```python
from build123d import *

# Parameters (mm, degrees)
BOSS_EXTRUDE1_DEPTH = 10
CUT_EXTRUDE1_DEPTH  = 10
SKETCH3_R           = 2.5
CUT_EXTRUDE2_DEPTH  = 7


with BuildPart() as part:
    # Sketch1 → Boss-Extrude1 (new body)
    with BuildSketch(Plane(origin=(0, 0, 0), x_dir=(1, 0, 0), z_dir=(0, 1, 0))):
        with BuildLine():
            Line((-40, 50), (40, 50))
            ThreePointArc((40, 50), (47.071067812, 47.071067812), (50, 40))
            Line((50, 40), (50, -40))
            ThreePointArc((50, -40), (47.071067812, -47.071067812), (40, -50))
            Line((40, -50), (-40, -50))
            ThreePointArc((-40, -50), (-47.071067812, -47.071067812), (-50, -40))
            Line((-50, -40), (-50, 40))
            ThreePointArc((-50, 40), (-47.071067812, 47.071067812), (-40, 50))
        make_face()
    extrude(amount=BOSS_EXTRUDE1_DEPTH)

    # Sketch2 → Cut-Extrude1 (cut)
    with BuildSketch(Plane(origin=(0, 10, 0), x_dir=(1, 0, 0), z_dir=(0, 1, 0))):
        with BuildLine():
            Line((-30, -40), (30, -40))
            ThreePointArc((30, -40), (37.071067812, -37.071067812), (40, -30))
            Line((40, -30), (40, 30))
            ThreePointArc((40, 30), (37.071067812, 37.071067812), (30, 40))
            Line((30, 40), (-30, 40))
            ThreePointArc((-30, 40), (-37.071067812, 37.071067812), (-40, 30))
            Line((-40, 30), (-40, -30))
            ThreePointArc((-40, -30), (-37.071067812, -37.071067812), (-30, -40))
        make_face()
    extrude(amount=-CUT_EXTRUDE1_DEPTH, mode=Mode.SUBTRACT)

    # Sketch3 → Cut-Extrude2 (cut)
    with BuildSketch(Plane(origin=(0, 10, 0), x_dir=(1, 0, 0), z_dir=(0, 1, 0))):
        with Locations(Location((-42, 42, 0), (0, 0, 270))):
            Circle(SKETCH3_R)
        with Locations(Location((42, 42, 0), (0, 0, 270))):
            Circle(SKETCH3_R)
        with Locations(Location((42.000013816, -42, 0), (0, 0, 270))):
            Circle(SKETCH3_R)
        with Locations(Location((-41.999986184, -42, 0), (0, 0, 270))):
            Circle(SKETCH3_R)
    extrude(amount=-CUT_EXTRUDE2_DEPTH, mode=Mode.SUBTRACT)


solid = part.part
```
Input: part model. Units: mm. Frame: model coordinates. A direction names the side the tool comes from. Coordinates: 2 decimals unless noted, no trailing zeros. Loops run counter-clockwise (first coordinate to the right, second up) from the corner with the lowest first, then second, coordinate; pieces in that order, holes last. Notation, with made-up numbers: M 36.25,-39.5 L 91.25,-39.5 A29 ccw 91.25,-19.5 Z; hole C 87.5,21.5 d6. An arc over 180 degrees is marked long. Use a Markdown table: item, result. Add a question column.
1) Section B-B, the plane z = -6.5. Return the cut outline in (x, y).
2) Section A-A, the plane x = -10.5. Return the cut outline in (y, z).
3) Pin query (flat end, axial travel): P1, Ø1.5, axis at x = 41, z = 42, coming from the +Y side; P2, Ø1, axis at x = 18.5, z = -38, coming from the -Y side. Return the tip coordinate at first contact, or that it passes through.
4) Section C-C, the plane y = 8. Return the cut outline in (x, z).
5) Section D-D, the plane z = -43. Return the cut outline in (x, y), plus the area to 3 significant figures.
6) Line query: L1, parallel to Z at x = -29, y = 9.25; L2, parallel to X at y = 4.75, z = -42. Output: solid intervals per line, ascending. Write a range as from..to.
7) Draft query along X for faces 4 (the cylindrical face through (-47.15, 4.93, -46.99)), 5 (the cylindrical face through (46.99, 4.93, -47.15)), 6 (the flat face through (1, 5, 50)), 7 (the flat face through (40, 5, 0)). Return one class per face: +X half, -X half, draft (parallel to the pull), parting line (faces both ways), or undercut.
8) Set-up query: faces 1 (the flat face through (0, 5, -40)), 2 (the flat face through (-50, 5, 1)), 3 (the cylindrical face through (41.04, 6.55, 44.31)). Return all of +Z, -Z, +X, -X, +Y, -Y with unobstructed straight access to the full face (end or side cutting, diameter ignored); none if empty.
Answer below:
| question | item | result |
|---|---|---|
| 1 | outline | M -50,0 L -40,0 L -40,10 L -50,10 Z; M 40,0 L 50,0 L 50,10 L 40,10 Z |
| 2 | outline | M 0,-50 L 10,-50 L 10,-40 L 0,-40 Z; M 0,40 L 10,40 L 10,50 L 0,50 Z |
| 3 | P1 | y = 3 |
| 3 | P2 | through |
| 4 | outline | M -50,-40 A10 ccw -40,-50 L 40,-50 A10 ccw 50,-40 L 50,40 A10 ccw 40,50 L -40,50 A10 ccw -50,40 Z; hole C -42,-42 d5; hole C -42,42 d5; hole M -40,-30 A10 ccw -30,-40 L 30,-40 A10 ccw 40,-30 L 40,30 A10 ccw 30,40 L -30,40 A10 ccw -40,30 Z; hole C 42,-42 d5; hole C 42,42 d5 |
| 5 | outline | M -49.54,0 L 49.54,0 L 49.54,10 L 44.29,10 L 44.29,3 L 39.71,3 L 39.71,10 L -39.71,10 L -39.71,3 L -44.29,3 L -44.29,10 L -49.54,10 Z |
| 5 | area | 927 mm2 |
| 6 | L1 | -50..-40, 40..50 |
| 6 | L2 | -49.8..-44.5, -39.5..39.5, 44.5..49.8 |
| 7 | face 4 | -X half |
| 7 | face 5 | +X half |
| 7 | face 6 | draft |
| 7 | face 7 | undercut |
| 8 | face 1 | +Y, -Y |
| 8 | face 2 | +Z, -Z, -X, +Y, -Y |
| 8 | face 3 | +Y |
